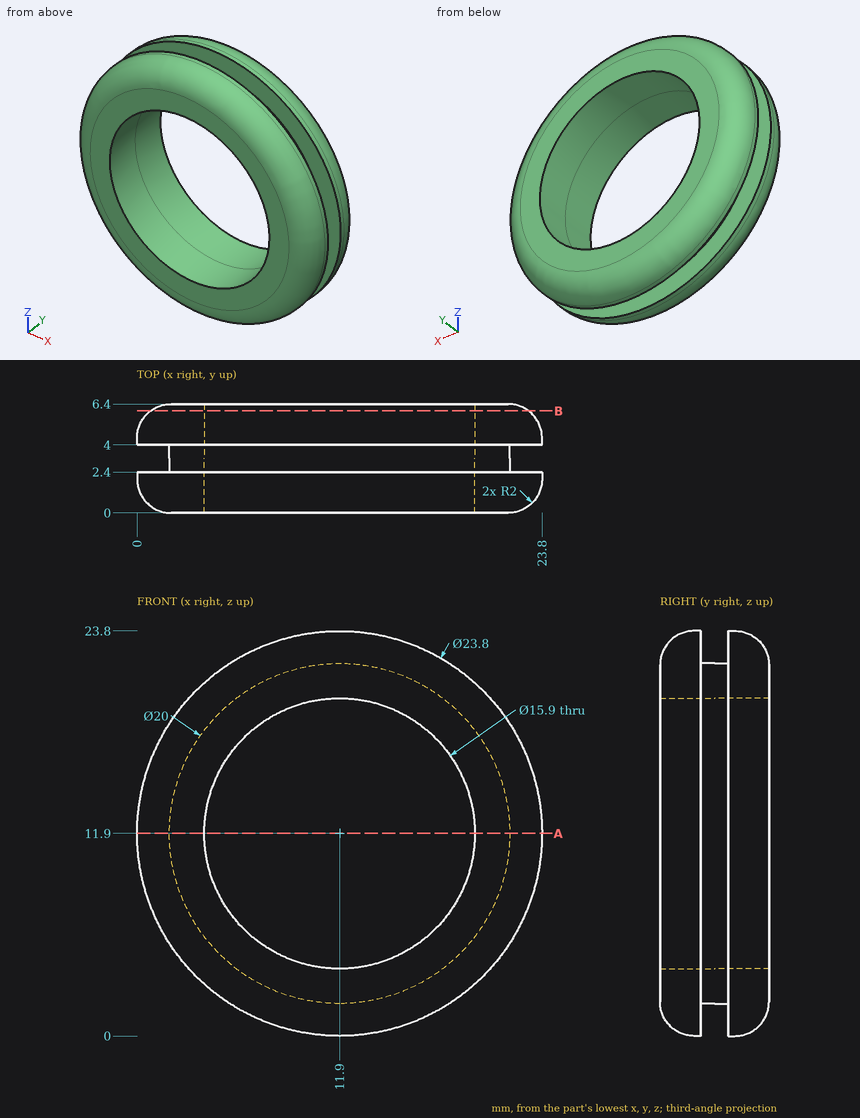
Geometry: see drawing. Coordinates: mm, zero at the bounding-box minimum. Round coordinates to 2 decimals unless told otherwise and drop trailing zeros. Loops run counter-clockwise (first coordinate to the right, second up) from the corner with the lowest first, then second, coordinate; pieces in that order, holes last. Notation, with made-up numbers: (79.25, -34.75) -> (95.25, -34.75) arc R27 cw to (95.25, 1.25) -> close; hole circle Ø9 at (-18, 56.5). An arc over 180 degrees is marked (long way). Write each question's results on one line, items separated by ' | '.
Item 1: Line query: probe 1 along X at (y, z) = (3.95, 11.9); probe 2 along X at (y, z) = (4.2, 11.9); probe 3 along Z at (x, y) = (11, 0.5). Output: solid intervals per line, ascending. Write a range as [from, to].
Answers below:
probe 1: x = [1.9, 3.95], [19.85, 21.9] | probe 2: x = [0, 3.95], [19.85, 23.8] | probe 3: z = [0.71, 4], [19.8, 23.09]
Item 2: Cut plane A-A on z = 11.9. Return the cut outline in (x, y), and give its area (3 significant figures).
Answers below:
outline: (0, 2) arc R2 ccw to (2, 0) -> (3.95, 0) -> (3.95, 6.4) -> (2, 6.4) arc R2 ccw to (0, 4.4) -> (0, 4) -> (1.9, 4) -> (1.9, 2.4) -> (0, 2.4) -> close; (19.85, 0) -> (21.8, 0) arc R2 ccw to (23.8, 2) -> (23.8, 2.4) -> (21.9, 2.4) -> (21.9, 4) -> (23.8, 4) -> (23.8, 4.4) arc R2 ccw to (21.8, 6.4) -> (19.85, 6.4) -> close | area: 41.0 mm²
Item 3: Cut plane B-B on y = 6. Return the cut outline in (x, z).
Answers below:
outline: circle Ø22.2 at (11.9, 11.9); hole circle Ø15.9 at (11.9, 11.9)
Item 4: Pin query (flat end, axial travel): pin 1 Ø1 at (y, z) = (1, 9) entering from -X; pin 2 Ø2 at (y, z) = (5.5, 4.5) entering from +X; pin 3 Ø2 at (y, z) = (5, 10) entering from -X. Return the tip coordinate at first contact, or that it passes through.
Answers below:
pin 1: stops at x = 0.38 | pin 2: stops at x = 21.74 | pin 3: stops at x = 0.05
